Input: part model. Units: mm. Frame: model coordinates. Face numbers are marked on the shaded views. A direction names the side the tool comes from. Coordinates: 2 decimals unless noted, no trailing zeros. Loops run counter-clockwise (first coordinate to the right, second up) from the corner with the lowest first, then second, coordinate; pieces in that order, holes last. Notation, with made-up numbers: (77.25, 32.5) - (87.25, 32.5) arc R25 ccw to (87.25, 44.5) - close; hole circle Ø11 at (74, 34.25). An arc over 180 degrees is marked (long way). Use a Markdown table: item, result. Add a question column.
1. Ray query, L1, parallel to Y at x = 0, z = 5.4; L2, parallel to Y at x = 0, z = 8.5; L3, parallel to X at y = 1.75, z = 1.25. Return the intervals inside material, ascending. Write a range as [from, to].
2. Access query for the marked faces 1, 2 and 3. Directions: +Z, -Z, +X, -X, +Y, -Y. A direction counts if a zero-diameter tool reaches every point of the face in a straight line with its end or side. Return the directions, or none.
3. Contact query for flat-ended pins moving along their axis: P1, Ø3, axis at x = 0, y = 0, coming from the +Z side; P2, Ø6.5, axis at x = 0, y = 1, coming from the -Z side. Output: stop coordinate, or through.
4. Section query A-A on x = 0. Return the cut outline in (y, z), then the cut area to 3 significant figures.
5. Section query C-C on y = -0.5. Return the cut outline in (x, z), then the cut area to 3 significant figures.
6. Section query D-D on z = 11.5. Return the cut outline in (x, y).
7. Draft query along Y for the marked faces 4, 5, 6 and 7. Return one class per face: released by +Y, released by -Y, zero draft, split by the parting line, or undercut.
8. Section query B-B on z = 1.5. Return the cut outline in (x, y), then the cut area to 3 significant figures.
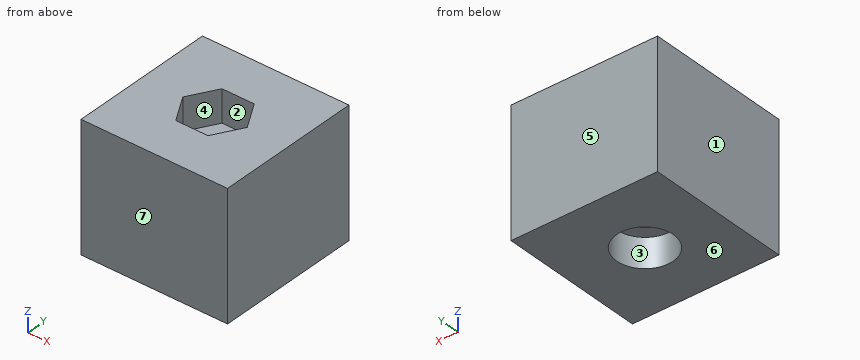
```python
from build123d import *

# Parameters (mm, degrees)
F0_W     = 15
F0_H     = 15
F0_R     = 2.9
F0_R_2   = 1.55
F0_R_3   = 1.35
F1_DEPTH = 13
F2_DEPTH = 8
F3_DEPTH = 3
F4_R     = 1.35
F5_DEPTH = 3.3


with BuildPart() as f1:
    # F0 (on Top) → F1 (new body)
    with BuildSketch(Plane.XY):
        Rectangle(F0_W, F0_H)
        Circle(F0_R, mode=Mode.SUBTRACT)
        Circle(F0_R)
        Circle(F0_R_2, mode=Mode.SUBTRACT)
        Circle(F0_R_2)
        Circle(F0_R_3, mode=Mode.SUBTRACT)
    extrude(amount=F1_DEPTH)

    # F0 (on Top) → F2 (cut)
    with BuildSketch(Plane.XY):
        Circle(F0_R_2)
        Circle(F0_R_3, mode=Mode.SUBTRACT)
    extrude(amount=F2_DEPTH, mode=Mode.SUBTRACT)

    # F0 (on Top) → F3 (cut)
    with BuildSketch(Plane.XY):
        Circle(F0_R)
        Circle(F0_R_2, mode=Mode.SUBTRACT)
    extrude(amount=F3_DEPTH, mode=Mode.SUBTRACT)

    # F4 (on face) → F5 (cut)
    with BuildSketch(Plane.XY.offset(13)):
        Polygon((3.3, 0), (1.65, 2.857884), (-1.65, 2.857884), (-3.3, 0), (-1.65, -2.857884), (1.65, -2.857884), align=None)
        Circle(F4_R, mode=Mode.SUBTRACT)
    extrude(amount=-F5_DEPTH, mode=Mode.SUBTRACT)


solid = f1.part
```
Resolved:
| question | item | result |
|---|---|---|
| 1 | L1 | [-7.5, -1.55], [1.55, 7.5] |
| 1 | L2 | [-7.5, -1.35], [1.35, 7.5] |
| 1 | L3 | [-7.5, -2.31], [2.31, 7.5] |
| 2 | face 1 | +Z, -Z, -X, +Y, -Y |
| 2 | face 2 | +Z |
| 2 | face 3 | -Z |
| 3 | P1 | z = 9.7 |
| 3 | P2 | z = 0 |
| 4 | outline | (-7.5, 0) - (-2.9, 0) - (-2.9, 3) - (-1.55, 3) - (-1.55, 8) - (-1.35, 8) - (-1.35, 9.7) - (-2.86, 9.7) - (-2.86, 13) - (-7.5, 13) - close; (1.35, 8) - (1.55, 8) - (1.55, 3) - (2.9, 3) - (2.9, 0) - (7.5, 0) - (7.5, 13) - (2.86, 13) - (2.86, 9.7) - (1.35, 9.7) - close |
| 4 | area | 139 mm² |
| 5 | outline | (-7.5, 0) - (-2.86, 0) - (-2.86, 3) - (-1.47, 3) - (-1.47, 8) - (-1.25, 8) - (-1.25, 9.7) - (-3.01, 9.7) - (-3.01, 13) - (-7.5, 13) - close; (1.25, 8) - (1.47, 8) - (1.47, 3) - (2.86, 3) - (2.86, 0) - (7.5, 0) - (7.5, 13) - (3.01, 13) - (3.01, 9.7) - (1.25, 9.7) - close |
| 5 | area | 139 mm² |
| 6 | outline | (-7.5, -7.5) - (7.5, -7.5) - (7.5, 7.5) - (-7.5, 7.5) - close; hole (-3.3, 0) - (-1.65, -2.86) - (1.65, -2.86) - (3.3, 0) - (1.65, 2.86) - (-1.65, 2.86) - close |
| 7 | face 4 | undercut |
| 7 | face 5 | released by +Y |
| 7 | face 6 | zero draft |
| 7 | face 7 | released by -Y |
| 8 | outline | (-7.5, -7.5) - (7.5, -7.5) - (7.5, 7.5) - (-7.5, 7.5) - close; hole circle Ø5.8 at (0, 0) |
| 8 | area | 199 mm² |
